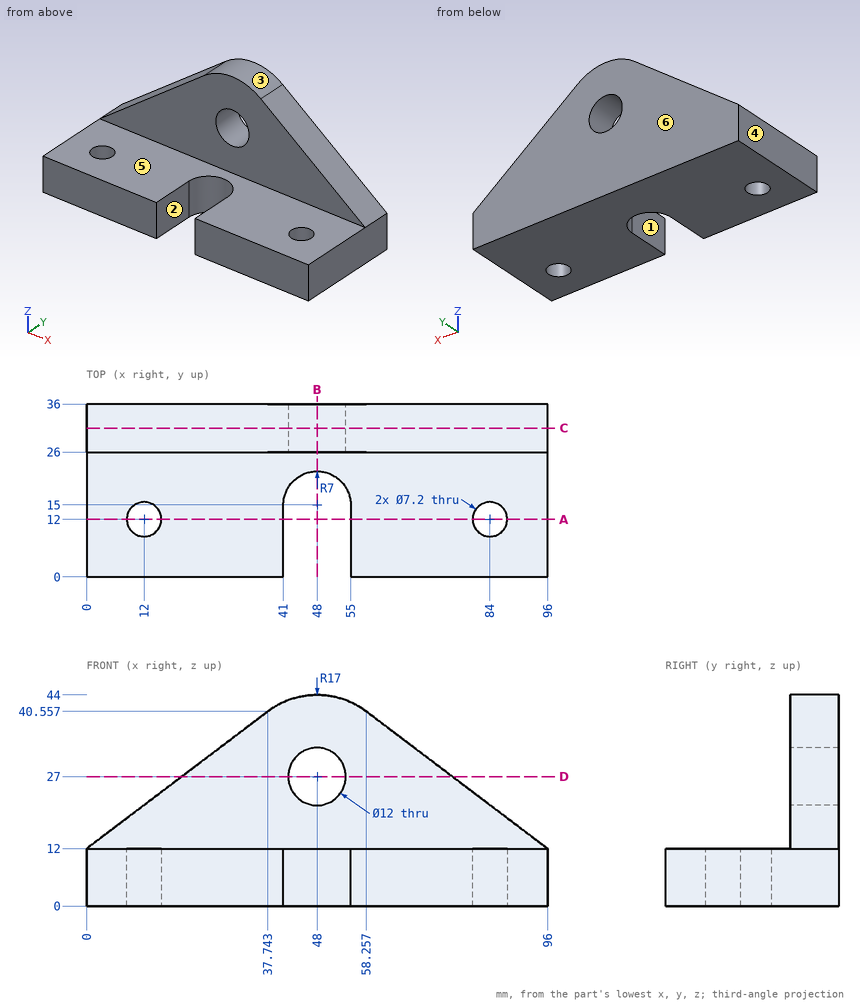
Print and shaded views of the part. All mm, measured from the part's lowest x, y and z. A direction names the side the tool comes from. Give positions to 0.01 mm unless a question says otherwise; leave off trailing zeros. Loops run counter-clockwise (first coordinate to the right, second up) from the corner with the lowest first, then second, coordinate; pieces in that order, holes last. Notation, with made-up numbers: (57.5, 39.25) -> (77.5, 39.25) arc R25 ccw to (77.5, 54.25) -> close; hole circle Ø10 at (46, -24). An arc over 180 degrees is marked (long way). Use a Markdown table: item, result.
1. Slice it at C-C (y = 31). List the corners of the cut face in (x, z).
Check result:
| item | result |
|---|---|
| outline | (0, 0) -> (96, 0) -> (96, 12) -> (58.26, 40.56) arc R17 ccw to (37.74, 40.56) -> (0, 12) -> close; hole circle Ø12 at (48, 27) |
2. Wall check: L1, parallel to Y at x = 84, z = 3.5; L2, parallel to X at y = 14, z = 3; L3, parallel to Z at x = 24, y = 4. Give the ranges that are in metal, low to high. Write a range as [from, to].
Check result:
| item | result |
|---|---|
| L1 | y = [0, 8.4], [15.6, 36] |
| L2 | x = [0, 9.01], [14.99, 41], [55, 81.01], [86.99, 96] |
| L3 | z = [0, 12] |
3. Flat gauge pins, fed straight in: pin 1 (16 mm diameter, centred on x = 53.5, z = 26, fed in from -Y); pin 2 (21 mm diameter, centred on x = 35, y = 7, fed in from +Z); pin 3 (6 mm diameter, centred on x = 25, y = 24, fed in from +Z). Where does each tip first touch, or does it go through?
Check result:
| item | result |
|---|---|
| pin 1 | stops at y = 26 |
| pin 2 | stops at z = 12 |
| pin 3 | stops at z = 32.61 |
4. Slice it at A-A (y = 12). List the corners of the cut face in (x, z), plus the area to 3 significant figures.
Check result:
| item | result |
|---|---|
| outline | (0, 0) -> (8.4, 0) -> (8.4, 12) -> (0, 12) -> close; (15.6, 0) -> (41, 0) -> (41, 12) -> (15.6, 12) -> close; (55, 0) -> (80.4, 0) -> (80.4, 12) -> (55, 12) -> close; (87.6, 0) -> (96, 0) -> (96, 12) -> (87.6, 12) -> close |
| area | 811 mm^2 |
5. Slice it at D-D (z = 27). List the corners of the cut face in (x, y) (1 decimal).
Check result:
| item | result |
|---|---|
| outline | (19.8, 26) -> (42, 26) -> (42, 36) -> (19.8, 36) -> close; (54, 26) -> (76.2, 26) -> (76.2, 36) -> (54, 36) -> close |
6. Which spindle directions (+Z, -Z, +X, -X, +Y, -Y) get a long thin tool onto all of the face, cutting with end or side? Do the marked faces 5 and 6. Say none if no direction does.
Check result:
| item | result |
|---|---|
| face 5 | +Z, +X, -X, -Y |
| face 6 | +Z, -Z, +X, -X, +Y |
7. Mould opens along X. For the marked faces 1, 2, 3 and 4 say: pulls with the +X half, pulls with the -X half, needs draft (parallel to the pull), parting line crosses it, or undercut.
Check result:
| item | result |
|---|---|
| face 1 | undercut |
| face 2 | undercut |
| face 3 | parting line crosses it |
| face 4 | pulls with the -X half |
8. Slice it at B-B (x = 48). List the corners of the cut face in (y, z).
Check result:
| item | result |
|---|---|
| outline | (22, 0) -> (36, 0) -> (36, 21) -> (26, 21) -> (26, 12) -> (22, 12) -> close; (26, 33) -> (36, 33) -> (36, 44) -> (26, 44) -> close |
